from build123d import *

# Parameters (mm, degrees)
SKETCH1_R           = 25
SKETCH1_R_2         = 10
BOSS_EXTRUDE1_DEPTH = 25
CUT_EXTRUDE1_DEPTH  = 2


with BuildPart() as part:
    # Sketch1 → Boss-Extrude1 (new body)
    with BuildSketch(Plane.XY):
        with BuildLine():
            Line((-5.9495669, 79.464935133), (-10.735337561, 40.593572422))
            ThreePointArc((-10.735337561, 40.593572422), (-13.846128401, 30.51133724), (-20.2552595, 22.12971899))
            ThreePointArc((-20.2552595, 22.12971899), (-27.455944575, 12.090124379), (-30, 0))
            Line((-30, 0), (-30, -30))
            Line((-30, -30), (30, -30))
            Line((30, -30), (30, 0))
            ThreePointArc((30, 0), (27.455944575, 12.090124379), (20.2552595, 22.12971899))
            ThreePointArc((20.2552595, 22.12971899), (13.846128401, 30.51133724), (10.735337561, 40.593572422))
            Line((10.735337561, 40.593572422), (5.9495669, 79.464935133))
            ThreePointArc((5.9495669, 79.464935133), (6.588547568, 84.397513141), (9.524776428, 88.412134191))
            ThreePointArc((9.524776428, 88.412134191), (14.000335083, 94.615706401), (14.834877403, 102.219552307))
            Line((14.834877403, 102.219552307), (22.415220632, 106.480398828))
            Line((22.415220632, 106.480398828), (17.935698756, 114.427937641))
            Line((17.935698756, 114.427937641), (10.795365576, 110.41441703))
            ThreePointArc((10.795365576, 110.41441703), (-11.019469666, 110.176997999), (-9.524776428, 88.412134191))
            ThreePointArc((-9.524776428, 88.412134191), (-6.588547568, 84.397513141), (-5.9495669, 79.464935133))
        make_face()
        Circle(SKETCH1_R, mode=Mode.SUBTRACT)
        with Locations((0, 100)):
            Circle(SKETCH1_R_2, mode=Mode.SUBTRACT)
    extrude(amount=BOSS_EXTRUDE1_DEPTH)

    # Sketch2 → Cut-Extrude1 (cut)
    with BuildSketch(Plane.XY.offset(25)):
        with BuildLine():
            Line((-2.424018912, 78.51885418), (-6.403368912, 32.676732655))
            ThreePointArc((-6.403368912, 32.676732655), (-3.537609758, 30.601194917), (0, 30.677021255))
            ThreePointArc((0, 30.677021255), (3.537609758, 30.601194917), (6.403368912, 32.676732655))
            Line((6.403368912, 32.676732655), (2.424018912, 78.51885418))
            ThreePointArc((2.424018912, 78.51885418), (0, 80.741469231), (-2.424018912, 78.51885418))
        make_face()
    extrude(amount=-CUT_EXTRUDE1_DEPTH, mode=Mode.SUBTRACT)


solid = part.part
Source: CAD feature listing. Evaluate the final solid. Frame: model axes, mm. A direction names the side the tool comes from. Give positions to 0.01 mm unless a question says otherwise; leave off trailing zeros. Order: outer loops, then holes, each group sorted by start corner. A loop starts at its lowest first (then second) coordinate and runs counter-clockwise, first axis right, second up. Notation, with made-up numbers: (-9.5, 45) -> (15.5, 45) arc R17 ccw to (15.5, 50) -> close; hole circle Ø4 at (-28, -8). An arc over 180 degrees is marked (long way). Write item = value, one per line.
Item 1: Section query C-C (y = 44). Output: boundary loops of the cut face in (x, z), then the cut area to 3 significant figures.
Check result:
outline = (-10.32, 0) -> (10.32, 0) -> (10.32, 25) -> (5.42, 25) -> (5.42, 23) -> (-5.42, 23) -> (-5.42, 25) -> (-10.32, 25) -> close
area = 494 mm²
Item 2: Section query A-A (z = 18.5). Output: boundary loops of the cut face in (x, y).
Check result:
outline = (-30, -30) -> (30, -30) -> (30, 0) arc R30 ccw to (20.26, 22.13) arc R30 cw to (10.74, 40.59) -> (5.95, 79.46) arc R10 cw to (9.52, 88.41) arc R15 ccw to (14.83, 102.22) -> (22.42, 106.48) -> (17.94, 114.43) -> (10.8, 110.41) arc R15 ccw (long way) to (-9.52, 88.41) arc R10 cw to (-5.95, 79.46) -> (-10.74, 40.59) arc R30 cw to (-20.26, 22.13) arc R30 ccw to (-30, 0) -> close; hole circle Ø50 at (0, 0); hole circle Ø20 at (0, 100)
Item 3: Section query D-D (x = 26.5). Output: boundary loops of the cut face in (y, z).
Check result:
outline = (-30, 0) -> (14.06, 0) -> (14.06, 25) -> (-30, 25) -> close
Item 4: Section query B-B (y = 100). Output: boundary loops of the cut face in (x, z), then the cut area to 3 significant figures.
Check result:
outline = (-15, 0) -> (-10, 0) -> (-10, 25) -> (-15, 25) -> close; (10, 0) -> (15, 0) -> (15, 25) -> (10, 25) -> close
area = 250 mm²
Item 5: Contact query for flat-ended pins moving along their axis: pin 1 (2 mm diameter, centred on y = 46.5, z = 9, fed in from -X); pin 2 (12 mm diameter, centred on y = 91.5, z = 9.5, fed in from +X); pin 3 (1.5 mm diameter, centred on y = 82.5, z = 17.5, fed in from +X). Output: stop coordinate, or through.
Check result:
pin_1 = -10.13
pin_2 = 14.79
pin_3 = 6.21
Item 6: Mould query, pull axis Y, two halves, no side actions, for faces 4 (the face through (30, -15, 12)), 5 (the face through (14.42, 112.45, 12.32)), 6 (the face through (0, -30, 12)), 7 (the face through (-8.31, 60.3, 12.32)). Classes: +Y half, -Y half, draft (parallel to the pull), parting line (faces both ways), or undercut.
Check result:
face_4 = draft
face_5 = +Y half
face_6 = -Y half
face_7 = undercut
Item 7: Ray query, probe 1 along Y at (x, z) = (0, 12); probe 2 along Y at (x, z) = (13, 18.75); probe 3 along X at (y, z) = (-10, 21). Return the intervals inside material, ascending.
Check result:
probe_1 = -30 to -25, 25 to 90, 110 to 115
probe_2 = -30 to -21.35, 21.35 to 32.29, 92.52 to 111.65
probe_3 = -30 to -22.91, 22.91 to 30
Item 8: Set-up query: faces 1 (the face through (23.846, 7.509, 12.325)), 2 (the face through (8.376, 59.757, 12.325)), 3 (the face through (-4.386, 55.919, 24.014)). Return all of +Z, -Z, +X, -X, +Y, -Y with unobstructed straight access to the full face (end or side cutting, diameter ignored); none if empty.
Check result:
face_1 = +Z, -Z
face_2 = +Z, -Z, +X
face_3 = +Z
